from build123d import *

# Parameters (mm, degrees)
SZKIC1_W                               = 24
SZKIC1_H                               = 8
WYTNIJ_WYCI_GNI_CIE1_REACH             = 10
SZKIC2_R                               = 4
WYTNIJ_WYCI_GNI_CIE1_DIRECTION_2_REACH = 10
SFAZOWANIE1_SIZE                       = 1


with BuildPart() as part:
    # Szkic1 → Obrót1 (revolve)
    with BuildSketch(Plane.XY):
        with Locations((12, 4)):
            Rectangle(SZKIC1_W, SZKIC1_H)
    revolve(axis=Axis((0, 0, 0), (1, 0, 0)))

    # Szkic2 → Wytnij-wyciągnięcie1 (cut, up to next)
    with BuildSketch(Plane(origin=(0, 0, 0), x_dir=(1, 0, 0), z_dir=(0, 1, 0)), mode=Mode.PRIVATE) as wytnij_wyci_gni_cie1_sk1:
        with Locations((12, 0)):
            Circle(SZKIC2_R)
    wytnij_wyci_gni_cie1_tool1 = extrude(wytnij_wyci_gni_cie1_sk1.sketch, amount=-WYTNIJ_WYCI_GNI_CIE1_REACH, mode=Mode.PRIVATE) & part.part
    add(wytnij_wyci_gni_cie1_tool1.solids().sort_by_distance((12, 0, 0))[0], mode=Mode.SUBTRACT)

    # Szkic2 → Wytnij-wyciągnięcie1 direction 2 (cut, up to next)
    with BuildSketch(Plane(origin=(0, 0, 0), x_dir=(1, 0, 0), z_dir=(0, 1, 0)), mode=Mode.PRIVATE) as wytnij_wyci_gni_cie1_direction_2_sk1:
        with Locations((12, 0)):
            Circle(SZKIC2_R)
    wytnij_wyci_gni_cie1_direction_2_tool1 = extrude(wytnij_wyci_gni_cie1_direction_2_sk1.sketch, amount=WYTNIJ_WYCI_GNI_CIE1_DIRECTION_2_REACH, mode=Mode.PRIVATE) & part.part
    add(wytnij_wyci_gni_cie1_direction_2_tool1.solids().sort_by_distance((12, 0, 0))[0], mode=Mode.SUBTRACT)

    # Sfazowanie1
    sfazowanie1_edges = [part.edges().sort_by_distance(p)[0] for p in [
        (0, -8, 0),
        (24, -8, 0),
    ]]
    chamfer(sfazowanie1_edges, length=SFAZOWANIE1_SIZE)


solid = part.part
Check sheet for the modelled part. Datum: model origin and axes. Units: mm. Round coordinates to 2 decimals unless told otherwise and drop trailing zeros. Loops run counter-clockwise (first coordinate to the right, second up) from the corner with the lowest first, then second, coordinate; pieces in that order, holes last. Notation, with made-up numbers: (55, 82.25) -> (70, 82.25) arc R18 cw to (70, 108.25) -> close; hole circle Ø5 at (26.25, 39). An arc over 180 degrees is marked (long way). Put each result on its own line as item: value. Start each with the question number.
1. Scan lines: probe 1 along X at (y, z) = (5.75, 0); probe 2 along X at (y, z) = (4, 1.5); probe 3 along Z at (x, y) = (13.5, 0.25). Record each from-to range of solid material in increasing order.
2. Section check B-B (x = 5.5). Enter the section's corners in (y, z).
3. Section check C-C (x = 12). Enter the section's corners in (y, z), plus the area to 3 significant figures.
4. Gauge pin test, flat ends, axial feed: pin 1 (1 mm diameter, centred on x = 3.5, z = 2.5, fed in from -Y); pin 2 (7 mm diameter, centred on x = 12, z = 0, fed in from +Y). Record the tip position at first contact, or that the pin passes through.
5. Section check A-A (z = 0). Enter the section's corners in (x, y).
Findings:
1. probe 1: x = 0 to 8, 16 to 24
1. probe 2: x = 0 to 8.29, 15.71 to 24
1. probe 3: z = -8 to -3.71, 3.71 to 8
2. outline: circle Ø16 at (0, 0)
3. outline: (-6.93, -4) arc R8 ccw to (6.93, -4) -> close; (-6.93, 4) -> (6.93, 4) arc R8 ccw to start
3. area: 78.6 mm^2
4. pin 1: stops at y = -7.75
4. pin 2: passes through
5. outline: (0, -7) -> (1, -8) -> (8, -8) -> (8, 8) -> (1, 8) -> (0, 7) -> close; (16, -8) -> (23, -8) -> (24, -7) -> (24, 7) -> (23, 8) -> (16, 8) -> close
